Model file for the job. Use its own axes, mm. A direction names the side the tool comes from. Round coordinates to 2 decimals unless told otherwise and drop trailing zeros. Order: outer loops, then holes, each group sorted by start corner. A loop starts at its lowest first (then second) coordinate and runs counter-clockwise, first axis right, second up. Notation, with made-up numbers: (44.25, -27) - (89.25, -27) arc R23 cw to (89.25, 4) - close; hole circle Ø2 at (24.25, -32). An arc over 180 degrees is marked (long way). Use one line per item in the form item = value.
from build123d import *

# Parameters (mm, degrees)
F1_DEPTH = 500.0625
F2_R     = 4.7625
F3_DEPTH = 6.351


with BuildPart() as f1:
    # F0 (on Front) → F1 (new body, symmetric)
    with BuildSketch(Plane.XZ):
        Polygon((0, 50.8), (0, 0), (50.8, 0), (50.8, 6.35), (6.35, 6.35), (6.35, 50.8), align=None)
    extrude(amount=F1_DEPTH, both=True)

    # F2 (on face) → F3 (cut, through all)
    with BuildSketch(Plane.XY.offset(6.35)):
        with Locations((28.575, 473.075)):
            Circle(F2_R)
        with Locations((28.575, 438.15)):
            Circle(F2_R)
        with Locations((28.575, 403.225)):
            Circle(F2_R)
        with Locations((28.575, 368.3)):
            Circle(F2_R)
        with Locations((28.575, 333.375)):
            Circle(F2_R)
        with Locations((28.575, 298.45)):
            Circle(F2_R)
        with Locations((28.575, 263.525)):
            Circle(F2_R)
        with Locations((28.575, 228.6)):
            Circle(F2_R)
        with Locations((28.575, 193.675)):
            Circle(F2_R)
        with Locations((28.575, 158.75)):
            Circle(F2_R)
        with Locations((28.575, -158.75)):
            Circle(F2_R)
        with Locations((28.575, -193.675)):
            Circle(F2_R)
        with Locations((28.575, -228.6)):
            Circle(F2_R)
        with Locations((28.575, -263.525)):
            Circle(F2_R)
        with Locations((28.575, -298.45)):
            Circle(F2_R)
        with Locations((28.575, -333.375)):
            Circle(F2_R)
        with Locations((28.575, -473.075)):
            Circle(F2_R)
        with Locations((28.575, -438.15)):
            Circle(F2_R)
        with Locations((28.575, -403.225)):
            Circle(F2_R)
        with Locations((28.575, -368.3)):
            Circle(F2_R)
    extrude(amount=-F3_DEPTH, mode=Mode.SUBTRACT)


solid = f1.part
(1) Tool access for faces 1 (the face through (25, -7, 0)), 2 (the face through (6.35, -7, 28)): list every direction of +Z, -Z, +X, -X, +Y, -Y with a clear straight run to the whole face (end or side of a thin tool).
Report:
face_1 = -Z, +X, -X, +Y, -Y
face_2 = +Z, +X, +Y, -Y
(2) Pin check, flat tips, straight feed: pin 1 (8.5 mm diameter, centred on x = 28.575, y = 473.075, fed in from -Z); pin 2 (10 mm diameter, centred on y = -123, z = 30.5, fed in from -X); pin 3 (12.5 mm diameter, centred on x = 28.575, y = -333.375, fed in from +Z); pin 4 (3 mm diameter, centred on y = -358, z = 9, fed in from +X). Stop position of each tip, or through.
Report:
pin_1 = through
pin_2 = 0
pin_3 = 6.35
pin_4 = 6.35
(3) Slice it at B-B on z = 20. Give the cut face in (x, y).
Report:
outline = (0, -500.06) - (6.35, -500.06) - (6.35, 500.06) - (0, 500.06) - close
(4) Slice it at C-C on x = 15.5. Give the cut face in (y, z).
Report:
outline = (-500.06, 0) - (500.06, 0) - (500.06, 6.35) - (-500.06, 6.35) - close
(5) Slice it at A-A on y = -137. Give the cut face in (x, z), then the cut area to 3 significant figures.
Report:
outline = (0, 0) - (50.8, 0) - (50.8, 6.35) - (6.35, 6.35) - (6.35, 50.8) - (0, 50.8) - close
area = 605 mm2
(6) Probe probe 1 along X at (y, z) = (-85, 27.5); probe 2 along X at (y, z) = (438.15, 2.25). List the from-to ranges inside material, lowest first. Write a range as [from, to].
Report:
probe_1 = [0, 6.35]
probe_2 = [0, 23.81], [33.34, 50.8]
